Part model, mm, in its own coordinate system. A direction names the side the tool comes from. Give positions to 0.01 mm unless a question says otherwise; leave off trailing zeros. Order: outer loops, then holes, each group sorted by start corner. A loop starts at its lowest first (then second) coordinate and runs counter-clockwise, first axis right, second up. Notation, with made-up numbers: M 70.5,40 L 84.5,40 A10 cw 84.5,55 Z; hole C -6.5,84.5 d2. An arc over 180 degrees is marked long. Return JSON: item names as keys, results as strings.
from build123d import *

# Parameters (mm, degrees)
F0_W          = 63.5
F0_H          = 63.5
F0_W_2        = 50.8
F0_H_2        = 50.8
F1_DEPTH      = 42.5
F1_DEPTH_BACK = 42.5
F3_D          = 4.4
F3_DEPTH      = 14.1
F3_TIP        = 1.3218933619
F5_D          = 28.575
F5_DEPTH      = 10
F5_TIP        = 8.5847960944
F7_D          = 6.6
F7_DEPTH      = 10
F7_TIP        = 1.9828400428
F9_D          = 18
F9_DEPTH      = 10
F9_TIP        = 5.4077455712


with BuildPart() as f1:
    # F0 (on Right) → F1 (new body, two sides)
    with BuildSketch(Plane.YZ) as f1_sk:
        Rectangle(F0_W, F0_H)
        Rectangle(F0_W_2, F0_H_2, mode=Mode.SUBTRACT)
    extrude(amount=F1_DEPTH)
    extrude(f1_sk.sketch, amount=-F1_DEPTH_BACK)

    # F3
    with Locations(Plane.XY.offset(31.75)):
        with Locations((-21.8, 0), (0, -21.8), (21.8, 0), (0, 21.8)):
            Hole(F3_D / 2, depth=F3_DEPTH)
            with Locations((0, 0, -(F3_DEPTH + F3_TIP / 2))):  # 118° drill point
                Cone(0, F3_D / 2, F3_TIP, mode=Mode.SUBTRACT)

    # F5
    with Locations(Plane.XY.offset(31.75)):
        with Locations((0, 0)):
            Hole(F5_D / 2, depth=F5_DEPTH)
            with Locations((0, 0, -(F5_DEPTH + F5_TIP / 2))):  # 118° drill point
                Cone(0, F5_D / 2, F5_TIP, mode=Mode.SUBTRACT)

    # F7
    with Locations(Plane(origin=(0, 0, -31.75), x_dir=(1, 0, 0), z_dir=(0, 0, -1))):
        with Locations((-17.5, -17.5), (-17.5, 17.5), (17.5, 17.5), (17.5, -17.5)):
            Hole(F7_D / 2, depth=F7_DEPTH)
            with Locations((0, 0, -(F7_DEPTH + F7_TIP / 2))):  # 118° drill point
                Cone(0, F7_D / 2, F7_TIP, mode=Mode.SUBTRACT)

    # F9
    with Locations(Plane(origin=(0, 0, -31.75), x_dir=(1, 0, 0), z_dir=(0, 0, -1))):
        with Locations((0, 0)):
            Hole(F9_D / 2, depth=F9_DEPTH)
            with Locations((0, 0, -(F9_DEPTH + F9_TIP / 2))):  # 118° drill point
                Cone(0, F9_D / 2, F9_TIP, mode=Mode.SUBTRACT)


solid = f1.part
Q1. Band-saw the part on D-D (y = 0). Give the cut face in (x, z), then the cut area to 3 significant figures.
Established:
{"outline": "M -42.5,-31.75 L -9,-31.75 L -9,-25.4 L -42.5,-25.4 Z; M -42.5,25.4 L -24,25.4 L -24,31.75 L -42.5,31.75 Z; M -19.6,25.4 L -14.29,25.4 L -14.29,31.75 L -19.6,31.75 Z; M 9,-31.75 L 42.5,-31.75 L 42.5,-25.4 L 9,-25.4 Z; M 14.29,25.4 L 19.6,25.4 L 19.6,31.75 L 14.29,31.75 Z; M 24,25.4 L 42.5,25.4 L 42.5,31.75 L 24,31.75 Z", "area": "728 mm²"}
Q2. Probe line 1 along Y through (x, z) = (0, 27.75); line 2 along X through (y, z) = (-17.5, -27); line 3 along Y through (x, z) = (-14.5, -22). List the from-to ranges inside material, lowest first.
Established:
{"line 1": "y = -31.75 to -24, -19.6 to -14.29, 14.29 to 19.6, 24 to 31.75", "line 2": "x = -42.5 to -20.8, -14.2 to 14.2, 20.8 to 42.5", "line 3": "y = -31.75 to -25.4, 25.4 to 31.75"}
Q3. Band-saw the part on A-A (z = 14.5). Give the cut face in (x, y).
Established:
{"outline": "M -42.5,-31.75 L 42.5,-31.75 L 42.5,-25.4 L -42.5,-25.4 Z; M -42.5,25.4 L 42.5,25.4 L 42.5,31.75 L -42.5,31.75 Z"}
Q4. Band-saw the part on B-B (x = 0). Give the cut face in (y, z), then the cut area to 3 significant figures.
Established:
{"outline": "M -31.75,-31.75 L -9,-31.75 L -9,-25.4 L -25.4,-25.4 L -25.4,25.4 L -24,25.4 L -24,31.75 L -31.75,31.75 Z; M -19.6,25.4 L -14.29,25.4 L -14.29,31.75 L -19.6,31.75 Z; M 9,-31.75 L 31.75,-31.75 L 31.75,31.75 L 24,31.75 L 24,25.4 L 25.4,25.4 L 25.4,-25.4 L 9,-25.4 Z; M 14.29,25.4 L 19.6,25.4 L 19.6,31.75 L 14.29,31.75 Z", "area": "1,100 mm²"}
Q5. 3-axis set-ups, long thin cutter, end or side, ignore diameter. For faces 4 (the cylindrical face through (20.8, 17.4, -28.5)), 5 (the flat face through (10, 0, -31.75)), 6 (the flat face through (1, 31.75, 0)), 7 (the cylindrical face through (0, 24, 29)), 8 (the flat face through (10, -12, 25.4)): which of +Z, -Z, +X, -X, +Y, -Y reach the whole face in a straight line?
Established:
{"face 4": "-Z", "face 5": "-Z, +X, -X, +Y, -Y", "face 6": "+Z, -Z, +X, -X, +Y", "face 7": "+Z", "face 8": "+X, -X"}
Q6. Pin check, flat tips, straight feed: pin 1 (1.5 mm diameter, centred on x = -15, y = 16, fed in from -Z); pin 2 (6 mm diameter, centred on x = 1, y = 7, fed in from +Z); pin 3 (16 mm diameter, centred on x = 0, y = 0, fed in from -Z); pin 4 (4 mm diameter, centred on x = -17.5, y = 17.5, fed in from -Z). Stop position of each tip, or through.
Established:
{"pin 1": "stops at z = -31.75", "pin 2": "stops at z = -25.4", "pin 3": "passes through", "pin 4": "stops at z = 25.4"}
Q7. Band-saw the part on C-C (y = -17.5). Give the cut face in (x, z), then the cut area to 3 significant figures.
Established:
{"outline": "M -42.5,-31.75 L -20.8,-31.75 L -20.8,-25.4 L -42.5,-25.4 Z; M -42.5,25.4 L 42.5,25.4 L 42.5,31.75 L -42.5,31.75 Z; M -14.2,-31.75 L 14.2,-31.75 L 14.2,-25.4 L -14.2,-25.4 Z; M 20.8,-31.75 L 42.5,-31.75 L 42.5,-25.4 L 20.8,-25.4 Z", "area": "996 mm²"}
Q8. Two-plate mould, pull along X, no slides. Class faces 1 (the cylindrical face through (-22.983, 1.855, 28.531)), 2 (the flat face through (1, -31.75, 0)), 3 (the flat face through (-42.5, -29, 0)): +X half, -X half, draft (parallel to the pull), parting line (faces both ways), or undercut.
Established:
{"face 1": "undercut", "face 2": "draft", "face 3": "-X half"}
